Job drawing, mm, ordinate dimensions from the low corner. One solid piece. Round coordinates to 2 decimals unless told otherwise and drop trailing zeros. Loops run counter-clockwise (first coordinate to the right, second up) from the corner with the lowest first, then second, coordinate; pieces in that order, holes last.
1) Mould opens along Z. For the marked faces 1 and 2 say: +Z half, -Z half, draft (parallel to the pull), parting line (faces both ways), or undercut.
2) Band-saw the part on B-B, the plane z = 35. Write the cut outline in (x, y), then the cut area to 3 significant figures.
3) Drop flat-ended pins along their axis: P1, Ø3, axis at x = 2, z = 11, coming from the +Y side; P2, Ø1, axis at y = 1, z = 8, coming from the -X side. Give the stop position or say it passes through.
4) Band-saw the part on D-D, the plane x = 0.5. Write the cut outline in (y, z) (1 decimal).
5) Band-saw the part on C-C, the plane y = 1.8. Write the cut outline in (x, z).
6) Band-saw the part on A-A, the plane x = 5.2. Write the cut outline in (y, z).
7) Probe line 1 (Z direction, x = 5.25, y = 1.8); line 2 (Z direction, x = 4.25, y = 2.1) (1 decimal); line 3 (Y direction, x = 6, z = 27.5). List the from-to ranges inside material, lowest first.
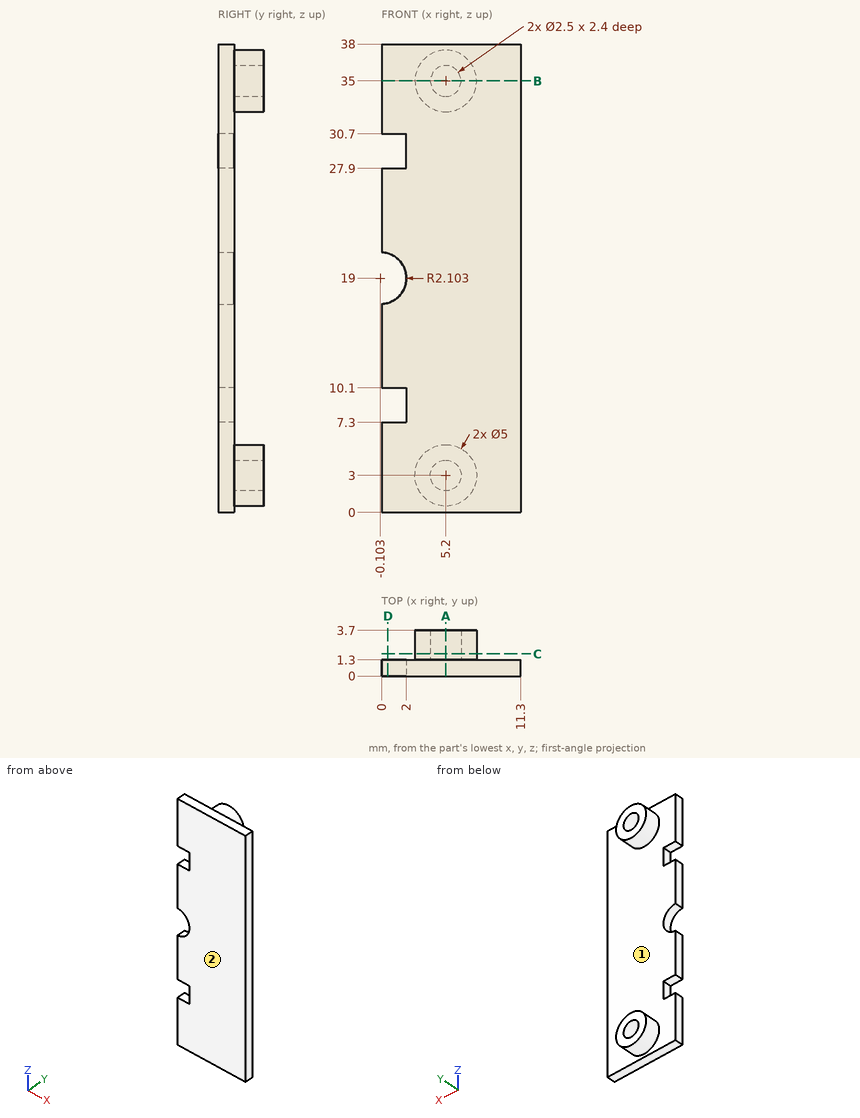
Reported:
1. face 1: undercut
1. face 2: draft
2. outline: (0, 0) - (11.3, 0) - (11.3, 1.3) - (7.7, 1.3) - (7.7, 3.7) - (6.45, 3.7) - (6.45, 1.3) - (3.95, 1.3) - (3.95, 3.7) - (2.7, 3.7) - (2.7, 1.3) - (0, 1.3) - close
2. area: 20.7 mm2
3. P1: stops at y = 1.3
3. P2: stops at x = 2
4. outline: (0, 0) - (1.3, 0) - (1.3, 7.3) - (0, 7.3) - close; (0, 10.1) - (1.3, 10.1) - (1.3, 17) - (0, 17) - close; (0, 21) - (1.3, 21) - (1.3, 27.9) - (0, 27.9) - close; (0, 30.7) - (1.3, 30.7) - (1.3, 38) - (0, 38) - close
5. outline: circle Ø5 at (5.2, 3); circle Ø5 at (5.2, 35); hole circle Ø2.5 at (5.2, 3); hole circle Ø2.5 at (5.2, 35)
6. outline: (0, 0) - (1.3, 0) - (1.3, 0.5) - (3.7, 0.5) - (3.7, 1.75) - (1.3, 1.75) - (1.3, 4.25) - (3.7, 4.25) - (3.7, 5.5) - (1.3, 5.5) - (1.3, 32.5) - (3.7, 32.5) - (3.7, 33.75) - (1.3, 33.75) - (1.3, 36.25) - (3.7, 36.25) - (3.7, 37.5) - (1.3, 37.5) - (1.3, 38) - (0, 38) - close
7. line 1: z = 0.5 to 1.75, 4.25 to 5.5, 32.5 to 33.75, 36.25 to 37.5
7. line 2: z = 0.7 to 2.2, 3.8 to 5.3, 32.7 to 34.2, 35.8 to 37.3
7. line 3: y = 0 to 1.3
